from build123d import *

# Parameters (mm, degrees)
BOSS_EXTRUDE1_DEPTH      = 1.85
BOSS_EXTRUDE1_DEPTH_BACK = 2
SKETCH1_R                = 2
SKETCH3_W                = 30
SKETCH3_H                = 10
BOSS_EXTRUDE3_DEPTH      = 7
SKETCH7_W                = 10
SKETCH7_H                = 5
BOSS_EXTRUDE7_DEPTH      = 2
FILLET2_R                = 2
SKETCH9_R                = 2
CUT_EXTRUDE3_DEPTH       = 10
FILLET3_R                = 1


with BuildPart() as part:
    # Sketch1 → Boss-Extrude1 (new, two sides: drawn at the far end of the back side and taken through both)
    with BuildSketch(Plane(origin=(0, 0, 0), x_dir=(1, 0, 0), z_dir=(0, 1, 0)).offset(-BOSS_EXTRUDE1_DEPTH_BACK)):
        with Locations(Location((0, 0, 0), (0, 0, 270))):
            Circle(SKETCH1_R)
    extrude(amount=BOSS_EXTRUDE1_DEPTH + BOSS_EXTRUDE1_DEPTH_BACK)

    # Sketch3 → Boss-Extrude3 (add)
    with BuildSketch(Plane(origin=(0, 1.85, 0), x_dir=(1, 0, 0), z_dir=(0, 1, 0))):
        Rectangle(SKETCH3_W, SKETCH3_H)
    extrude(amount=BOSS_EXTRUDE3_DEPTH)

    # Sketch7 → Boss-Extrude7 (add)
    with BuildSketch(Plane.XZ.offset(2)):
        Rectangle(SKETCH7_W, SKETCH7_H)
    extrude(amount=-BOSS_EXTRUDE7_DEPTH)

    # Fillet2
    fillet2_edges = [part.edges().sort_by_distance(p)[0] for p in [
        (5, -1, 2.5),
        (5, -1, -2.5),
        (-5, -1, -2.5),
        (-5, -1, 2.5),
    ]]
    fillet(fillet2_edges, radius=FILLET2_R)

    # Sketch9 → Cut-Extrude3 (cut)
    with BuildSketch(Plane(origin=(0, 0, -5), x_dir=(-1, 0, 0), z_dir=(0, 0, -1))):
        with Locations((-11, 5.35)):
            Circle(SKETCH9_R)
        with Locations((11, 5.35)):
            Circle(SKETCH9_R)
    extrude(amount=-CUT_EXTRUDE3_DEPTH, mode=Mode.SUBTRACT)

    # Fillet3
    fillet3_edges = [part.edges().sort_by_distance(p)[0] for p in [
        (-15, 5.35, 5),
        (15, 8.85, 0),
        (0, 8.85, -5),
        (-15, 8.85, 0),
        (0, 8.85, 5),
        (15, 1.85, 0),
        (15, 5.35, 5),
        (0, 1.85, -5),
        (15, 5.35, -5),
        (-15, 1.85, 0),
        (-15, 5.35, -5),
        (0, 1.85, 5),
    ]]
    fillet(fillet3_edges, radius=FILLET3_R)


solid = part.part
Can you work these out from the model? Positions are in its coordinate system, mm. A direction names the side the tool comes from. Round coordinates to 2 decimals unless told otherwise and drop trailing zeros. Write each loop counter-clockwise with the first axis right and the second up, starting at its lowest first coordinate (ties: lowest second). Pieces come first, ordered by that corner, then holes. Notation, with made-up numbers: (-32.5, 3.25) - (-6.5, 3.25) arc R24 cw to (-6.5, 18.25) - close; hole circle Ø4 at (-8.5, 2). An arc over 180 degrees is marked (long way). Write each question's results on one line, items separated by ' | '. Start each with the question number.
1) Suppose I cut it at A-A (y = 3.75). List the corners of the cut face in (x, z) for me.
2) Suppose I cut it at B-B (x = -11). List the corners of the cut face in (y, z) for me.
3) Which directions (+Z, -Z, +X, -X, +Y, -Y) give clear straight access to the entire face, cutting with the end or side of a thin tool? Please do faces 1 (the cylindrical face through (4.4, -0.99, -1.93)), 2 (the cylindrical face through (-4.43, -0.99, 1.9)), 3 (the flat face through (-5, -1, 0)).
4) Please list where these lines run through material, in increasing order: line 1 (Y direction, x = 11, z = 3.25); line 2 (X direction, y = 6.75, z = -2.5); line 3 (X direction, y = 4.5, z = -4.5).
5) Suppose I cut it at C-C (z = 0). List the corners of the cut face in (x, y) for me.
6) Suppose I cut it at D-D (x = 8.5). List the corners of the cut face in (y, z) for me, and give its area (3 significant figures).
7) For pin 1 Ø0.5 at (y, z) = (-1, 0) entering from +X; pin 2 Ø1 at (x, y) = (1, -1) entering from -Z; pin 3 Ø1.5 at (x, y) = (-5.5, -1) entering from -Z, each with a flat end and sliding along its axis, tell me the tip position at first contact or that it passes through.
8) We'd pull the mould along X, two halves only. Please class faces 4 (the flat face through (0, -1, 2.5)), 5 (the cylindrical face through (-9.413, 4.133, -0.07)), 6 (the cylindrical face through (-2, 1, 0)): released by +X, released by -X, zero draft, split by the parting line, or undercut.
Here are the results:
1) outline: (-15, -4) arc R1 ccw to (-14, -5) - (-12.2, -5) - (-12.2, 5) - (-14, 5) arc R1 ccw to (-15, 4) - close; (-9.8, -5) - (9.8, -5) - (9.8, 5) - (-9.8, 5) - close; (12.2, -5) - (14, -5) arc R1 ccw to (15, -4) - (15, 4) arc R1 ccw to (14, 5) - (12.2, 5) - close
2) outline: (1.85, -4) arc R1 ccw to (2.85, -5) - (3.35, -5) - (3.35, 5) - (2.85, 5) arc R1 ccw to (1.85, 4) - close; (7.35, -5) - (7.85, -5) arc R1 ccw to (8.85, -4) - (8.85, 4) arc R1 ccw to (7.85, 5) - (7.35, 5) - close
3) face 1: -Z, +X, -Y | face 2: +Z, -X, -Y | face 3: +Z, -Z, -X, -Y
4) line 1: y = 1.85 to 3.35, 7.35 to 8.85 | line 2: x = -15 to -12.43, -9.57 to 9.57, 12.43 to 15 | line 3: x = -14.87 to -12.81, -9.19 to 9.19, 12.81 to 14.87
5) outline: (-15, 2.85) arc R1 ccw to (-14, 1.85) - (-2, 1.85) - (-2, 0) - (-5, 0) - (-5, -2) - (5, -2) - (5, 0) - (2, 0) - (2, 1.85) - (14, 1.85) arc R1 ccw to (15, 2.85) - (15, 7.85) arc R1 ccw to (14, 8.85) - (-14, 8.85) arc R1 ccw to (-15, 7.85) - close; hole circle Ø4 at (-11, 5.35); hole circle Ø4 at (11, 5.35)
6) outline: (1.85, -4) arc R1 ccw to (2.85, -5) - (7.85, -5) arc R1 ccw to (8.85, -4) - (8.85, 4) arc R1 ccw to (7.85, 5) - (2.85, 5) arc R1 ccw to (1.85, 4) - close | area: 69.1 mm2
7) pin 1: stops at x = 5 | pin 2: stops at z = -2.5 | pin 3: stops at z = -1.47
8) face 4: zero draft | face 5: undercut | face 6: split by the parting line
